The listing builds one solid part. Answer for the finished solid, in the listing's coordinates (mm). Face numbers are marked on the shaded views. A direction names the side the tool comes from. Give positions to 0.01 mm unless a question says otherwise; leave off trailing zeros. Write each loop counter-clockwise with the first axis right and the second up, starting at its lowest first coordinate (ties: lowest second). Pieces come first, ordered by that corner, then holes. Notation, with made-up numbers: (85.5, 44.5) - (140.5, 44.5) arc R19 cw to (140.5, 69.5) - close; hole circle Ø1 at (17, 74.25). An arc over 180 degrees is marked (long way). One line per question, with ' | ' between items. Start each with the question number.
1. A cutting plane is placed at B-B (z = 65). Determine the outline of the cut face in (x, y).
2. The mould has two halves that part along X. Classify the marked faces 5, 6 and 7: +X half, -X half, draft (parallel to the pull), parting line (faces both ways), or undercut.
3. A cutting plane is placed at A-A (y = 84.5). Determine the outline of the cut face in (x, z), then the cut area to 3 significant figures.
4. A cutting plane is placed at C-C (y = -4.5). Determine the outline of the cut face in (x, z), then the cut area to 3 significant figures.
5. For the marked faces 1, 2, 3 and 4, determine the directions among +Z, -Z, +X, -X, +Y, -Y from which every point of the face is accessible in a straight line to the end or side of a thin tool.
6. Given P1, Ø12, axis at x = 28, y = 93, coming from the +Z side; P2, Ø6.5, axis at x = -12.5, z = 5, coming from the -Y side; P3, Ø5, axis at x = -12.5, z = 5, coming from the +Y side; P4, Ø8, axis at x = -41, z = -27.5, coming from the +Y side, each flat-ended and moving along its own axis, determine where each tip first touches the part or whether it passes through.
7. Find the intervals of material crossed by L1, parallel to X at y = 162, z = -18.5; L2, parallel to X at y = 132, z = 5; L3, parallel to X at y = 138.5, z = 5, in increasing order. Write a range as from..to.
```python
from build123d import *

# Parameters (mm, degrees)
SKICA4_R                    = 4
ODEBRAT_VYSUNUT_M1_DEPTH    = 161.15617378
SKICA5_R                    = 9
SKICA5_R_2                  = 4
P_IDAT_VYSUNUT_M1_DEPTH     = 1.5
SKICA6_W                    = 90
SKICA6_H                    = 10
P_IDAT_VYSUNUT_M3_DEPTH     = 53
ODEBRAT_VYSUNUT_M2_DEPTH    = 35
SKICA7_R                    = 25
ODEBRAT_VYSUNUT_M3_DEPTH    = 173.081696102
SKICA9_W                    = 47
SKICA9_H                    = 81.822124963
ODEBRAT_VYSUNUT_M4_DEPTH    = 216.313980348
M6_Z_VIT1_D                 = 5
M6_Z_VIT1_DEPTH             = 17
M6_Z_VIT1_CSINK_D           = 6.05
M6_Z_VIT1_CSINK_ANGLE       = 90
M6_Z_VIT1_TIP               = 1.502151548
P_IDAT_START                = -53
P_IDAT_VYSUNUT_M4_DEPTH     = 106
SKICA14_W                   = 78
SKICA14_H                   = 70
ODEBRAT_VYSUNUT_M5_DEPTH    = 30
SKICA15_R                   = 4
ODEBRAT_VYSUNUT_M6_DEPTH    = 208.347197072
SKICA16_W                   = 80
SKICA16_H                   = 4
P_IDAT_VYSUNUT_M5_DEPTH     = 1
ZKOSEN_4_SIZE               = 3
ZKOSEN_2_SIZE               = 15
ZKOSEN_2_SIZE2              = 25.980762114
ZKOSEN_3_SIZE               = 3
M10X1_25_Z_VIT1_D           = 8.8
M10X1_25_Z_VIT1_DEPTH       = 26.25
M10X1_25_Z_VIT1_CSINK_D     = 10.05
M10X1_25_Z_VIT1_CSINK_ANGLE = 90
M10X1_25_Z_VIT1_TIP         = 2.643786724
ODEBRAT_VYSUNUT_M7_REACH    = 217.754
SKICA25_R                   = 4
SKICA26_R                   = 9
SKICA26_R_2                 = 2
P_IDAT_VYSUNUT_M6_DEPTH     = 6


# Read off the part's stored shape, not the designer's step: P_idat vysunut_m4, M6 z_vit2
with BuildPart() as part:
    # Skica2 → Rotovat1 (revolve)
    with BuildSketch(Plane.XY, mode=Mode.PRIVATE) as rotovat1_sk:
        Polygon((25, 0), (45, 0), (45, 10), (33, 10), (33, 18), (56.428571429, 18), (56.428571429, 26), (33, 26), (33, 34), (67.857142857, 34), (67.857142857, 42), (33, 42), (33, 50), (73.571428571, 50), (73.571428571, 58), (33, 58), (33, 66), (75, 66), (75, 74), (33, 74), (33, 82), (75, 82), (75, 90), (33, 90), (33, 98), (75, 98), (75, 106), (33, 106), (33, 114), (75, 114), (75, 122), (40, 122), (40, 140), (0, 140), (0, 120), (25, 120), align=None)
    revolve(rotovat1_sk.sketch.rotate(Axis((0, 148.651800879, 0), (0, -1, 0)), 90), axis=Axis((0, 148.651800879, 0), (0, -1, 0)))

    # Skica4 → Odebrat vysunut_m1 (cut, through all)
    with BuildSketch(Plane.XZ.offset(-120)):
        with Locations(Location((12.5, 5, 0), (0, 0, 270))):
            Circle(SKICA4_R)
        with Locations(Location((-12.5, 5, 0), (0, 0, 270))):
            Circle(SKICA4_R)
    extrude(amount=-ODEBRAT_VYSUNUT_M1_DEPTH, mode=Mode.SUBTRACT)

    # Skica5 → P_idat vysunut_m1 (add, symmetric)
    # profile 1 of 2: a face of its own
    with BuildSketch(Plane(origin=(0, 140, 0), x_dir=(1, 0, 0), z_dir=(0, 1, 0))):
        with Locations(Location((-12.5, -5, 0), (0, 0, 90))):
            Circle(SKICA5_R)
        with Locations(Location((-12.5, -5, 0), (0, 0, 90))):
            Circle(SKICA5_R_2, mode=Mode.SUBTRACT)
    # profile 2 of 2: a face of its own
    with BuildSketch(Plane(origin=(0, 140, 0), x_dir=(1, 0, 0), z_dir=(0, 1, 0))):
        with Locations(Location((12.5, -5, 0), (0, 0, 90))):
            Circle(SKICA5_R)
        with Locations(Location((12.5, -5, 0), (0, 0, 90))):
            Circle(SKICA5_R_2, mode=Mode.SUBTRACT)
    extrude(amount=P_IDAT_VYSUNUT_M1_DEPTH, both=True)

    # Skica6 → P_idat vysunut_m3 (add, symmetric)
    with BuildSketch(Plane(origin=(0, 0, 0), x_dir=(0, 0, -1), z_dir=(1, 0, 0))):
        with Locations((0, 5)):
            Rectangle(SKICA6_W, SKICA6_H)
        Polygon((-45, 0), (-45, 10), (-81.822124963, -23), (-81.822124963, -43), (-61.822124963, -43), (-36, 0), align=None)
        Polygon((36, 0), (-36, 0), (-61.822124963, -43), (61.822124963, -43), align=None)
        Polygon((81.822124963, -23), (45, 10), (45, 0), (36, 0), (61.822124963, -43), (81.822124963, -43), align=None)
    extrude(amount=P_IDAT_VYSUNUT_M3_DEPTH, both=True)

    # Skica6_5 → Odebrat vysunut_m2 (cut, symmetric)
    with BuildSketch(Plane(origin=(0, 0, 0), x_dir=(0, 0, -1), z_dir=(1, 0, 0))):
        Polygon((36, 0), (-36, 0), (-61.822124963, -43), (61.822124963, -43), align=None)
    extrude(amount=ODEBRAT_VYSUNUT_M2_DEPTH, both=True, mode=Mode.SUBTRACT)

    # Skica7 → Odebrat vysunut_m3 (cut, through all)
    with BuildSketch(Plane(origin=(0, 10, 0), x_dir=(1, 0, 0), z_dir=(0, 1, 0))):
        with Locations(Location((0, 0, 0), (0, 0, 270))):
            Circle(SKICA7_R)
    extrude(amount=-ODEBRAT_VYSUNUT_M3_DEPTH, mode=Mode.SUBTRACT)

    # Skica8 → Odebrat rotac_1 (revolve, cut)
    with BuildSketch(Plane.XZ.offset(43)):
        Polygon((-73, 0), (-73, 29), (-51, 29), (-51, 31), (51, 31), (51, 29), (73, 29), (73, 0), align=None)
    revolve(axis=Axis((-111.075378668, -43, 0), (1, 0, 0)), mode=Mode.SUBTRACT)

    # Skica9 → Odebrat vysunut_m4 (cut, through all)
    with BuildSketch(Plane.XZ.offset(43)):
        Polygon((-100, 81.822124963), (-100, 0), (-53, 0), (-53, 29), (-53, 81.822124963), align=None)
        with Locations((-76.5, -40.911062482)):
            Rectangle(SKICA9_W, SKICA9_H)
        with Locations((76.5, -40.911062482)):
            Rectangle(SKICA9_W, SKICA9_H)
        Polygon((53, 29), (53, 0), (100, 0), (100, 81.822124963), (53, 81.822124963), align=None)
    extrude(amount=-ODEBRAT_VYSUNUT_M4_DEPTH, mode=Mode.SUBTRACT)

    # M6 z_vit1
    with Locations(Plane(origin=(0, -43, 0), x_dir=(-1, 0, 0), z_dir=(0, -1, 0))):
        with Locations((-47, 46.822124963), (-25, 75.822124963), (25, -75.822124963), (47, -46.822124963), (25, 75.822124963), (-25, -75.822124963), (-47, -46.822124963), (47, 46.822124963)):
            CounterSinkHole(M6_Z_VIT1_D / 2, M6_Z_VIT1_CSINK_D / 2, depth=M6_Z_VIT1_DEPTH, counter_sink_angle=M6_Z_VIT1_CSINK_ANGLE)
            with Locations((0, 0, -(M6_Z_VIT1_DEPTH + M6_Z_VIT1_TIP / 2))):  # 118° drill point
                Cone(0, M6_Z_VIT1_D / 2, M6_Z_VIT1_TIP, mode=Mode.SUBTRACT)



with BuildPart() as body_2:
    # P_idat vysunut_m4 outline → P_idat vysunut_m4 (new body)
    with BuildSketch(Plane(origin=(0, 0, 0), x_dir=(0, 0, -1), z_dir=(1, 0, 0)).offset(P_IDAT_START)):
        Polygon((40, 140), (27, 170), (-40, 170), (-40, 122), (40, 122), align=None)
    extrude(amount=P_IDAT_VYSUNUT_M4_DEPTH)

    # Skica14 → Odebrat vysunut_m5 (cut)
    with BuildSketch(Plane(origin=(0, 170, 0), x_dir=(1, 0, 0), z_dir=(0, 1, 0))):
        with Locations((0, 5)):
            Rectangle(SKICA14_W, SKICA14_H)
    extrude(amount=-ODEBRAT_VYSUNUT_M5_DEPTH, mode=Mode.SUBTRACT)

    # Skica15 → Odebrat vysunut_m6 (cut, through all)
    with BuildSketch(Plane(origin=(0, 140, 0), x_dir=(1, 0, 0), z_dir=(0, 1, 0))):
        with Locations(Location((12.5, -5, 0), (0, 0, 90))):
            Circle(SKICA15_R)
        with Locations(Location((-12.5, -5, 0), (0, 0, 90))):
            Circle(SKICA15_R)
    extrude(amount=-ODEBRAT_VYSUNUT_M6_DEPTH, mode=Mode.SUBTRACT)


with BuildPart() as part_1:
    add(part.part)

    add(body_2.part)  # P_idat vysunut_m5 merges body 2
    # Skica16 → P_idat vysunut_m5 (add)
    with BuildSketch(Plane(origin=(53, 0, 0), x_dir=(0, 0, -1), z_dir=(1, 0, 0))):
        with Locations((0, 122)):
            Rectangle(SKICA16_W, SKICA16_H)
    extrude(amount=-P_IDAT_VYSUNUT_M5_DEPTH)

    # Zkosen_4
    zkosen_4_edges = [part_1.edges().sort_by_distance(p)[0] for p in [
        (-12.5, 120, 9),
        (12.5, 120, 9),
    ]]
    chamfer(zkosen_4_edges, length=ZKOSEN_4_SIZE)

    # Skica17 → Odebrat rotac_2 (revolve, cut)
    with BuildSketch(Plane(origin=(0, 0, 5), x_dir=(0, -1, 0), z_dir=(0, 0, 1))):
        Polygon((-170, 58), (-157, 58), (-157, 51), (-155, 51), (-155, -51), (-157, -51), (-157, -58), (-170, -58), align=None)
    revolve(axis=Axis((88.270190347, 170, 5), (-1, 0, 0)), mode=Mode.SUBTRACT)

    # M6 z_vit2 outline → M6 z_vit2 (revolve, cut)
    with BuildSketch(Plane(origin=(46, 0, -18.5), x_dir=(1, 0, 0), z_dir=(0, 0, 1))):
        Polygon((0, 170), (0, 151.497848452), (2.5, 153), (2.5, 169.475), (3.025, 170), align=None)
    revolve(axis=Axis((46, 0, -18.5), (0, 1, 0)), mode=Mode.SUBTRACT)

    # M6 z_vit2 2 outline → M6 z_vit2 2 (revolve, cut)
    with BuildSketch(Plane(origin=(-46, 0, 30), x_dir=(1, 0, 0), z_dir=(0, 0, 1))):
        Polygon((0, 170), (0, 151.497848452), (2.5, 153), (2.5, 169.475), (3.025, 170), align=None)
    revolve(axis=Axis((-46, 0, 30), (0, 1, 0)), mode=Mode.SUBTRACT)

    # M6 z_vit2 3 outline → M6 z_vit2 3 (revolve, cut)
    with BuildSketch(Plane(origin=(46, 0, 30), x_dir=(1, 0, 0), z_dir=(0, 0, 1))):
        Polygon((0, 170), (0, 151.497848452), (2.5, 153), (2.5, 169.475), (3.025, 170), align=None)
    revolve(axis=Axis((46, 0, 30), (0, 1, 0)), mode=Mode.SUBTRACT)

    # M6 z_vit2 4 outline → M6 z_vit2 4 (revolve, cut)
    with BuildSketch(Plane(origin=(-46, 0, -18.5), x_dir=(1, 0, 0), z_dir=(0, 0, 1))):
        Polygon((0, 170), (0, 151.497848452), (2.5, 153), (2.5, 169.475), (3.025, 170), align=None)
    revolve(axis=Axis((-46, 0, -18.5), (0, 1, 0)), mode=Mode.SUBTRACT)

    # Zkosen_2
    zkosen_2_edges = [part_1.edges().sort_by_distance(p)[0] for p in [
        (0, 140, -40),
    ]]
    zkosen_2_side = [part_1.faces().sort_by_distance(p)[0] for p in [
        (0, 131, -40),
    ]]
    chamfer(zkosen_2_edges, length=ZKOSEN_2_SIZE, length2=ZKOSEN_2_SIZE2, reference=zkosen_2_side[0])

    # Zkosen_3
    zkosen_3_edges = [part_1.edges().sort_by_distance(p)[0] for p in [
        (0, 120, -25),
    ]]
    chamfer(zkosen_3_edges, length=ZKOSEN_3_SIZE)

    # M10x1.25 z_vit1
    with Locations(Plane(origin=(0, 111.070508076, -64.126587737), x_dir=(1, 0, 0), z_dir=(0, 0.8660254037844383, -0.5000000000000007))):
        with Locations((0, -42.858983849)):
            CounterSinkHole(M10X1_25_Z_VIT1_D / 2, M10X1_25_Z_VIT1_CSINK_D / 2, depth=M10X1_25_Z_VIT1_DEPTH, counter_sink_angle=M10X1_25_Z_VIT1_CSINK_ANGLE)
            with Locations((0, 0, -(M10X1_25_Z_VIT1_DEPTH + M10X1_25_Z_VIT1_TIP / 2))):  # 118° drill point
                Cone(0, M10X1_25_Z_VIT1_D / 2, M10X1_25_Z_VIT1_TIP, mode=Mode.SUBTRACT)

    # Skica25 → Odebrat vysunut_m7 (cut, up to next)
    with BuildSketch(Plane.XY.offset(40), mode=Mode.PRIVATE) as odebrat_vysunut_m7_sk1:
        with Locations((-12.5, 131.5)):
            Circle(SKICA25_R)
    odebrat_vysunut_m7_tool1 = extrude(odebrat_vysunut_m7_sk1.sketch, amount=-ODEBRAT_VYSUNUT_M7_REACH, mode=Mode.PRIVATE) & part_1.part
    # Skica25 → Odebrat vysunut_m7 (cut, up to next)
    with BuildSketch(Plane.XY.offset(40), mode=Mode.PRIVATE) as odebrat_vysunut_m7_sk2:
        with Locations((12.5, 131.5)):
            Circle(SKICA25_R)
    odebrat_vysunut_m7_tool2 = extrude(odebrat_vysunut_m7_sk2.sketch, amount=-ODEBRAT_VYSUNUT_M7_REACH, mode=Mode.PRIVATE) & part_1.part
    add(odebrat_vysunut_m7_tool1.solids().sort_by_distance((-12.5, 131.5, 40))[0], mode=Mode.SUBTRACT)
    add(odebrat_vysunut_m7_tool2.solids().sort_by_distance((12.5, 131.5, 40))[0], mode=Mode.SUBTRACT)

    # Skica26 → P_idat vysunut_m6 (add)
    # profile 1 of 2: a face of its own
    with BuildSketch(Plane(origin=(0, 141.5, 0), x_dir=(1, 0, 0), z_dir=(0, 1, 0))):
        with Locations(Location((-12.5, -5, 0), (0, 0, 90))):
            Circle(SKICA26_R)
        with Locations(Location((-12.5, -5, 0), (0, 0, 270))):
            Circle(SKICA26_R_2, mode=Mode.SUBTRACT)
    # profile 2 of 2: a face of its own
    with BuildSketch(Plane(origin=(0, 141.5, 0), x_dir=(1, 0, 0), z_dir=(0, 1, 0))):
        with Locations(Location((12.5, -5, 0), (0, 0, 90))):
            Circle(SKICA26_R)
        with Locations(Location((12.5, -5, 0), (0, 0, 270))):
            Circle(SKICA26_R_2, mode=Mode.SUBTRACT)
    extrude(amount=-P_IDAT_VYSUNUT_M6_DEPTH)


solid = part_1.part
```
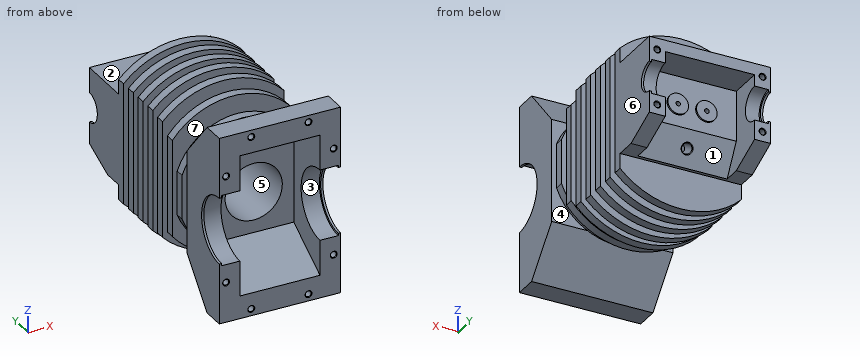
Determined:
1) outline: (-53, -43) - (53, -43) - (53, -7.92) - (-53, -7.92) - close; (-37.42, 66) - (37.42, 66) - (37.42, 74) - (-37.42, 74) - close; (-37.42, 82) - (37.42, 82) - (37.42, 90) - (-37.42, 90) - close; (-37.42, 98) - (37.42, 98) - (37.42, 106) - (-37.42, 106) - close; (-37.42, 114) - (37.42, 114) - (37.42, 122) - (-37.42, 122) - close; (-34.46, 50) - (34.46, 50) - (34.46, 58) - (-34.46, 58) - close; (-19.48, 34) - (19.48, 34) - (19.48, 42) - (-19.48, 42) - close
2) face 5: undercut | face 6: +X half | face 7: draft
3) outline: (-53, -53.07) arc R75 ccw to (53, -53.07) - (53, 53.07) arc R75 ccw to (-53, 53.07) - close; hole circle Ø50 at (0, 0) | area: 12,500 mm2
4) outline: (-53, -61.18) - (53, -61.18) - (53, 61.18) - (-53, 61.18) - close; hole (-35, -38.7) - (35, -38.7) - (35, 38.7) - (-35, 38.7) - close | area: 7,550 mm2
5) face 1: -Z, +Y | face 2: +Z, +X, -X, +Y | face 3: -Y | face 4: none
6) P1: z = 71.45 | P2: y = 135.5 | P3: y = 141.5 | P4: y = 170
7) L1: -53..-48.5, -43.5..-39, 39..43.5, 48.5..53 | L2: -53..-16.5, -8.5..8.5, 16.5..53 | L3: -53..-14.5, -10.5..10.5, 14.5..53
